from build123d import *

# Parameters (mm, degrees)
SKETCH2_W           = 200
SKETCH2_H           = 350
BOSS_EXTRUDE1_DEPTH = 100
CUT_EXTRUDE3_DEPTH  = 226
SKETCH5_W           = 97.727308895
SKETCH5_H           = 31.680459025
CUT_EXTRUDE4_DEPTH  = 284.94541729
SCALE1_SCALE        = 0.35


with BuildPart() as part:
    # Sketch2 → Boss-Extrude1 (new body)
    with BuildSketch(Plane(origin=(0, 0, 0), x_dir=(1, 0, 0), z_dir=(0, 1, 0))):
        Rectangle(SKETCH2_W, SKETCH2_H)
    extrude(amount=BOSS_EXTRUDE1_DEPTH)

    # Sketch4 → Cut-Extrude3 (cut, through all)
    with BuildSketch(Plane(origin=(0, 100, 0), x_dir=(1, 0, 0), z_dir=(0, 1, 0))):
        with BuildLine():
            Line((100, 175), (43.347633031, 175))
            Line((43.347633031, 175), (43.347633031, 77.272691105))
            ThreePointArc((43.347633031, 77.272691105), (45.866803863, 67.555664213), (52.789694192, 60.286522394))
            ThreePointArc((52.789694192, 60.286522394), (87.404145859, 23.940813259), (100, -24.644321249))
            Line((100, -24.644321249), (100, 175))
        make_face()
        with BuildLine():
            Line((-43.347633031, 77.272691105), (-43.347633031, 175))
            Line((-43.347633031, 175), (-100, 175))
            Line((-100, 175), (-100, -24.644321206))
            ThreePointArc((-100, -24.644321206), (-87.404145849, 23.940813278), (-52.789694192, 60.286522394))
            ThreePointArc((-52.789694192, 60.286522394), (-45.866803863, 67.555664213), (-43.347633031, 77.272691105))
        make_face()
        with BuildLine():
            Line((60, -175), (60, -24.644321162))
            ThreePointArc((60, -24.644321162), (0, 35.355678838), (-60, -24.644321162))
            Line((-60, -24.644321162), (-60, -175))
            Line((-60, -175), (60, -175))
        make_face()
    extrude(amount=-CUT_EXTRUDE3_DEPTH, mode=Mode.SUBTRACT)

    # Sketch5 → Cut-Extrude4 (cut, through all)
    with BuildSketch(Plane(origin=(100, 0, 0), x_dir=(0, 0, -1), z_dir=(1, 0, 0))):
        with BuildLine():
            Line((-175, 100), (-175, 50))
            ThreePointArc((-175, 50), (-160.355339059, 85.355339059), (-125, 100))
            Line((-125, 100), (-175, 100))
        make_face()
        with BuildLine():
            ThreePointArc((-105, 50), (-125, 70), (-145, 50))
            Line((-145, 50), (-105, 50))
        make_face()
        with BuildLine():
            Line((-105, 50), (-145, 50))
            ThreePointArc((-145, 50), (-125, 30), (-105, 50))
        make_face()
        with BuildLine():
            ThreePointArc((-125, 0), (-160.355339059, 14.644660941), (-175, 50))
            Line((-175, 50), (-175, 0))
            Line((-175, 0), (-125, 0))
        make_face()
        with BuildLine():
            ThreePointArc((-83.15716493, 22.628899304), (-101.215078672, 6.019578022), (-125, 0))
            Line((-125, 0), (-24.644321162, 0))
            Line((-24.644321162, 0), (-24.644321162, 31.680459025))
            Line((-24.644321162, 31.680459025), (-66.420030902, 31.680459025))
            ThreePointArc((-66.420030902, 31.680459025), (-75.933999434, 29.272627817), (-83.15716493, 22.628899304))
        make_face()
        with BuildLine():
            Line((-124.644321162, 100), (-125, 100))
            ThreePointArc((-125, 100), (-101.215078672, 93.980421978), (-83.15716493, 77.371100696))
            ThreePointArc((-83.15716493, 77.371100696), (-75.933999434, 70.727372183), (-66.420030902, 68.319540975))
            Line((-66.420030902, 68.319540975), (-24.644321162, 68.319540975))
            Line((-24.644321162, 68.319540975), (-24.644321162, 100))
            Line((-24.644321162, 100), (-124.644321162, 100))
        make_face()
        Polygon((60.286522394, 100), (-24.644321162, 100), (-24.644321162, 68.319540975), (77.272691105, 68.319540975), (77.272691105, 100), align=None)
        Polygon((-24.644321162, 31.680459025), (-24.644321162, 0), (60.286522394, 0), (77.272691105, 0), (77.272691105, 31.680459025), align=None)
        with Locations((126.136345553, 15.840229513)):
            Rectangle(SKETCH5_W, SKETCH5_H)
        with Locations((126.136345553, 84.159770487)):
            Rectangle(SKETCH5_W, SKETCH5_H)
    extrude(amount=-CUT_EXTRUDE4_DEPTH, mode=Mode.SUBTRACT)


with BuildPart() as part_1:
    # Scale1: scaled about (0, 50, 16.903782196)
    add(part.part.scale(SCALE1_SCALE).moved(Location((0, 32.5, 10.987458427))))


solid = part_1.part
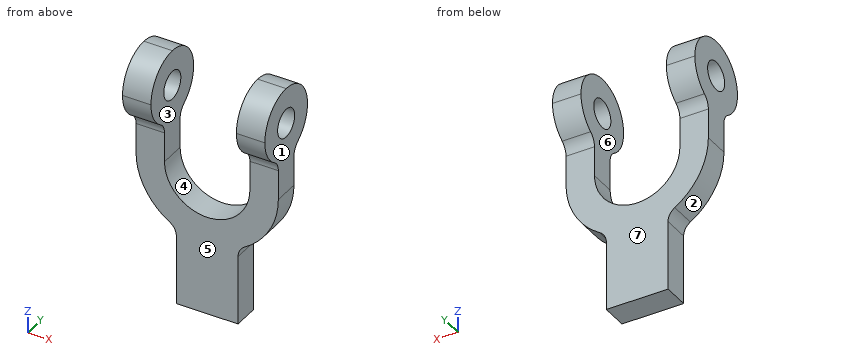
Check sheet for the modelled part. Datum: model origin and axes. Units: mm. Face numbers are marked on the shaded views. A direction names the side the tool comes from. Coordinates: 2 decimals unless noted, no trailing zeros. Write each loop counter-clockwise with the first axis right and the second up, starting at its lowest first coordinate (ties: lowest second). Pieces come first, ordered by that corner, then holes.
Item 1: Mould release check, pull along X, two halves, no side actions. Record for the marked faces 1, 2, 3 and 4: released by +X, released by -X, zero draft, split by the parting line, or undercut.
Numbers:
face 1: released by +X
face 2: released by -X
face 3: undercut
face 4: undercut
Item 2: Cross-section at C-C on y = 35. Record the boundary of the cut face in (x, z), then the cut area to 3 significant figures.
Numbers:
outline: (-35, 45.72) - (-21, 45.72) - (-21, 63.75) - (-35, 63.75) - close; (21, 45.72) - (35, 45.72) - (35, 63.75) - (21, 63.75) - close
area: 505 mm2
Item 3: Scan lines: probe 1 along X at (y, z) = (40, 45); probe 2 along Z at (x, y) = (-25, 50); probe 3 along Z at (x, y) = (26.5, 48.5). Record each from-to range of solid material in increasing order.
Numbers:
probe 1: x = -35 to -21, 21 to 35
probe 2: z = -4.88 to 47.74, 61.74 to 72.24
probe 3: z = -3.25 to 47.9, 61.57 to 72.17
Item 4: Access from +Z, -Z, +X, -X, +Y, -Y to the whole of each face (thin tool, end or side, straight path). Record for the marked faces 5, 6 and 7.
Numbers:
face 5: -Z, +X, -X, -Y
face 6: +Z, +Y, -Y
face 7: -Z, +X, -X, +Y
Item 5: Cross-section at B-B on x = 22.5. Record the boundary of the cut face in (y, z).
Numbers:
outline: (40.42, 40.09) arc R7 cw to (43.59, 34.23) - (43.59, -7.2) - (56.41, -7.2) - (56.41, 34.23) arc R7 cw to (59.58, 40.09) arc R17.5 ccw (long way) to start; hole circle Ø14 at (50, 54.74)
Item 6: Cross-section at D-D on z = 57.5. Record the boundary of the cut face in (x, y), then the cut area to 3 significant figures.
Numbers:
outline: (-35, 32.72) - (-21, 32.72) - (-21, 43.57) - (-35, 43.57) - close; (-35, 56.43) - (-21, 56.43) - (-21, 67.28) - (-35, 67.28) - close; (21, 32.72) - (35, 32.72) - (35, 43.57) - (21, 43.57) - close; (21, 56.43) - (35, 56.43) - (35, 67.28) - (21, 67.28) - close
area: 608 mm2
Item 7: Depth check by flat-ended pin: pin 1 Ø12 at (y, z) = (58.5, 11) entering from -X; pin 2 Ø12 at (y, z) = (58.5, 9.5) entering from -X; pin 3 Ø18 at (y, z) = (50, 54.74) entering from -X; pin 4 Ø6.5 at (y, z) = (52.5, -32) entering from -X. Enter the tip coordinate at first touch or a pass-through.
Numbers:
pin 1: stops at x = -34.87
pin 2: stops at x = -34.71
pin 3: stops at x = -35
pin 4: stops at x = -15.17
Item 8: Cross-section at A-A on z = 1.5. Record the boundary of the cut face in (x, y).
Numbers:
outline: (-29.95, 43.59) - (-10.63, 43.59) - (-10.63, 56.41) - (-29.95, 56.41) - close; (10.63, 43.59) - (29.95, 43.59) - (29.95, 56.41) - (10.63, 56.41) - close
